Design review of the part built by this model. Coordinates are the model's own, in mm. Round coordinates to 2 decimals unless told otherwise and drop trailing zeros. Order: outer loops, then holes, each group sorted by start corner. A loop starts at its lowest first (then second) coordinate and runs counter-clockwise, first axis right, second up. Notation, with made-up numbers: (25.25, -11.75) - (47.25, -11.75) arc R8 ccw to (47.25, -1.75) - close; hole circle Ø9 at (65.5, 69.25). An arc over 180 degrees is marked (long way). Use CSV: the item, a comma, the result in double quotes.
from build123d import *

# Parameters (mm, degrees)
SKETCH1_R               = 11
SKETCH1_R_2             = 9.5
BOSS_EXTRUDE1_DEPTH     = 95.5
CUT_EXTRUDE1_DEPTH      = 12
CUT_EXTRUDE1_DEPTH_BACK = 12


with BuildPart() as part:
    # Sketch1 → Boss-Extrude1 (new body)
    with BuildSketch(Plane(origin=(0, 0, 0), x_dir=(1, 0, 0), z_dir=(0, 1, 0))):
        Circle(SKETCH1_R)
        Circle(SKETCH1_R_2, mode=Mode.SUBTRACT)
    extrude(amount=BOSS_EXTRUDE1_DEPTH)

    # Sketch2 → Cut-Extrude1 (cut, two sides)
    with BuildSketch(Plane.XY) as cut_extrude1_sk:
        with BuildLine():
            ThreePointArc((-7, 83), (-6.121320344, 85.121320344), (-4, 86))
            Line((-4, 86), (4, 86))
            ThreePointArc((4, 86), (6.121320344, 85.121320344), (7, 83))
            Line((7, 83), (7, 22))
            ThreePointArc((7, 22), (6.121320344, 19.878679656), (4, 19))
            Line((4, 19), (-4, 19))
            ThreePointArc((-4, 19), (-6.121320344, 19.878679656), (-7, 22))
            Line((-7, 22), (-7, 83))
        make_face()
    extrude(amount=CUT_EXTRUDE1_DEPTH, mode=Mode.SUBTRACT)
    extrude(cut_extrude1_sk.sketch, amount=-CUT_EXTRUDE1_DEPTH_BACK, mode=Mode.SUBTRACT)


solid = part.part
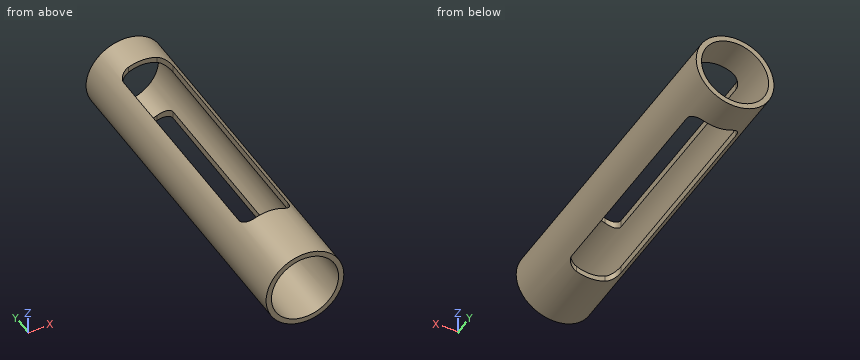
1) To check wall thickness, follow L1, parallel to Y at x = 1.25, z = 10.25; L2, parallel to X at y = 76, z = 0; L3, parallel to X at y = 58.5, z = -1. State the ranges of each line that lie inside material, in increasing order. Write a range as from..to.
Data:
L1,"y = 0..19, 86..95.5"
L2,"x = -11..-9.5, 9.5..11"
L3,"x = -10.95..-9.45, 9.45..10.95"
2) We need section C-C (z = 0). Give the boundary of the cut face in (x, y), then the cut area to 4 significant figures.
Data:
outline,"(-11, 0) - (-9.5, 0) - (-9.5, 95.5) - (-11, 95.5) - close; (9.5, 0) - (11, 0) - (11, 95.5) - (9.5, 95.5) - close"
area,"286.5 mm2"
3) Insertion check: pin 1 Ø1 at (y, z) = (52, -7) entering from +X; pin 2 Ø1.5 at (x, y) = (7, 67.5) entering from +Z; pin 3 Ø1 at (y, z) = (26, 5.5) entering from +X; pin 4 Ø4 at (x, z) = (-0.5, 7) entering from +Y. Each pin has a flat end and moves straight along its axis. Give the tip position at first contact, or say it passes through.
Data:
pin 1,"stops at x = 8.87"
pin 2,"stops at z = 8.49"
pin 3,"stops at x = 9.8"
pin 4,"passes through"
4) We need section B-B (y = 51.5). Give the boundary of the cut face in (x, z).
Data:
outline,"(-7, -8.49) - (-7, -6.42) arc R9.5 cw to (-7, 6.42) - (-7, 8.49) arc R11 ccw to start; (7, -8.49) arc R11 ccw to (7, 8.49) - (7, 6.42) arc R9.5 cw to (7, -6.42) - close"
5) We need section A-A (x = 0). Give the boundary of the cut face in (y, z), then the cut area to 3 significant figures.
Data:
outline,"(0, -11) - (19, -11) - (19, -9.5) - (0, -9.5) - close; (0, 9.5) - (19, 9.5) - (19, 11) - (0, 11) - close; (86, -11) - (95.5, -11) - (95.5, -9.5) - (86, -9.5) - close; (86, 9.5) - (95.5, 9.5) - (95.5, 11) - (86, 11) - close"
area,"85.5 mm2"
6) We need section D-D (y = 88.5). Give the boundary of the cut face in (x, z), then the cut area to 3 significant figures.
Data:
outline,"circle Ø22 at (0, 0); hole circle Ø19 at (0, 0)"
area,"96.6 mm2"
